For this review, take the finished solid that the model builds, in its own axes (mm). A direction names the side the tool comes from. Round coordinates to 2 decimals unless told otherwise and drop trailing zeros. Loops run counter-clockwise (first coordinate to the right, second up) from the corner with the lowest first, then second, coordinate; pieces in that order, holes last. Notation, with made-up numbers: (76.25, 6) -> (122.25, 6) arc R22 cw to (122.25, 37) -> close; hole circle Ø4 at (-16.75, -18.75). An arc over 180 degrees is marked (long way). Write each question's results on one line, items separated by ' | '.
```python
from build123d import *

# Parameters (mm, degrees)
F1_DEPTH = 80
F2_R     = 12.7
F3_DEPTH = 80


with BuildPart() as f1:
    # F0 (on Front) → F1 (new body)
    with BuildSketch(Plane.XZ):
        Polygon((540.943911, 841.859221), (-52.497789, 0), (12.897508, -46.098321), (606.147254, 795.488594), align=None)
    extrude(amount=F1_DEPTH)

    # F2 (on face) → F3 (cut, through all)
    with BuildSketch(Plane.XZ.offset(80)):
        with Locations((550.496222, 785.975975)):
            Circle(F2_R)
    extrude(amount=-F3_DEPTH, mode=Mode.SUBTRACT)

    # F4: F1 across plane


with BuildPart() as f1_1:
    add(f1.part)
    add(f1.part.mirror(Plane.YZ))


solid = f1_1.part
```
1. Consider section A-A (z = 349). State the section outline as (x, y) points.
Values found:
outline: (-291.41, -80) -> (-193.52, -80) -> (-193.52, 0) -> (-291.41, 0) -> close; (193.52, -80) -> (291.41, -80) -> (291.41, 0) -> (193.52, 0) -> close
2. Tool access review of faces 1 (the face through (138, 0, 268)), 2 (the face through (274.26, -39.44, 463.54)): name each direction out of +Z, -Z, +X, -X, +Y, -Y from which nothing blocks a thin tool from reaching the whole face with its end or side.
Values found:
face 1: +Z, -Z, +X, -X, +Y | face 2: +Z, +Y, -Y
3. Consider section D-D (z = 57). State the section outline as (x, y) points.
Values found:
outline: (-85.57, -80) -> (85.57, -80) -> (85.57, 0) -> (-85.57, 0) -> close
4. Consider section C-C (x = -302.5). State the section outline as (y, z) points.
Values found:
outline: (-80, 364.73) -> (0, 364.73) -> (0, 503.6) -> (-80, 503.6) -> close
5. Consider section B-B (y = -51.5). State the section outline as (x, z) points (1 decimal).
Values found:
outline: (-606.1, 795.5) -> (-48.9, 5) -> (-52.5, 0) -> (-38.4, -10) -> (-12.9, -46.1) -> (0, -37) -> (12.9, -46.1) -> (38.4, -10) -> (52.5, 0) -> (48.9, 5) -> (606.1, 795.5) -> (540.9, 841.9) -> (0, 74.5) -> (-540.9, 841.9) -> close; hole circle Ø25.4 at (-550.5, 786); hole circle Ø25.4 at (550.5, 786)
6. Draft analysis for pull direction X (two halves, no side actions). For faces 3 (the face through (-274.26, -39.44, 463.54)), 4 (the face through (-574, -39.44, 818.35)), 5 (the face through (323.646, -39.44, 394.731)), state which applies: released by +X, released by -X, zero draft, split by the parting line, or undercut.
Values found:
face 3: undercut | face 4: released by -X | face 5: released by +X
7. For pin 1 (23 mm diameter, centred on x = -550.5, z = 785.98, fed in from +Y); pin 2 (12 mm diameter, centred on x = -274, y = -55.5, fed in from -Z); pin 3 (3 mm diameter, centred on x = -287.5, y = -9.5, fed in from +Z); pin 4 (1 mm diameter, centred on y = -27.5, z = 218, fed in from +X), all flat-tipped, find the tip position at first contact; note any pin that passes through.
Values found:
pin 1: passes through | pin 2: stops at z = 315.79 | pin 3: stops at z = 484.45 | pin 4: stops at x = 199.42
8. To check wall thickness, follow probe 1 along X at (y, z) = (-62, 679.5); probe 2 along X at (y, z) = (-40, 718); probe 3 along Z at (x, y) = (-231, -15.5). State the ranges of each line that lie inside material, in increasing order.
Values found:
probe 1: x = -524.38 to -426.49, 426.49 to 524.38 | probe 2: x = -551.52 to -453.63, 453.63 to 551.52 | probe 3: z = 263.3 to 402.17
